Could you check a few things on this model? Use its own coordinates, in mm. A direction names the side the tool comes from. Round coordinates to 2 decimals unless told otherwise and drop trailing zeros. Write each loop counter-clockwise with the first axis right and the second up, starting at its lowest first coordinate (ties: lowest second). Pieces come first, ordered by that corner, then holes. Notation, with made-up numbers: M 67.25,25 L 94.25,25 A14 cw 94.25,38 Z; hole C -39,86 d11. An arc over 180 degrees is marked long. One line per item, written item: value. Start each with the question number.
(1) I want a section at C-C on x = -10. Please give me the cut outline in (y, z), and give its area (3 significant figures).
(2) I want a section at D-D on y = 20. Please give me the cut outline in (x, z).
(3) I want a section at B-B on y = 0. Please give me the cut outline in (x, z), and give its area (3 significant figures).
(4) Thinking about a two-plate mould opening in Y: for faces 4 (the face through (31, 9.76, 49.3)), 5 (the face through (162.942, 0, 50)), 6 (the face through (-121.037, -5.42, 74.406)), which applies, released by +Y, released by -Y, zero draft, split by the parting line, or undercut?
(5) I want a section at A-A on z = 17. Please give me the cut outline in (x, y), and give its area (3 significant figures).
(6) I'm going to push flat-ended pins straight in: pin 1 Ø1 at (x, y) = (-8.5, -41.5) entering from -Z; pin 2 Ø5 at (y, z) = (44.5, 53) entering from +X; pin 3 Ø10 at (y, z) = (-47, 45.5) entering from -X; pin 4 Ø10 at (x, z) = (-54.5, 81.5) entering from +Y. Where does each tip first touch, or does it pass through?
(7) Which directions (+Z, -Z, +X, -X, +Y, -Y) give clear straight access to the entire face, cutting with the end or side of a thin tool? Please do faces 1 (the face through (-77.942, 11, 27)), 2 (the face through (119.847, -5.42, 25.594)), 3 (the face through (-39.517, -67.185, 49.3)).
(8) If I drill on L1, parallel to Y at x = 0, z = 68; L2, parallel to Z at x = -141, y = -5.5; L3, parallel to Y at x = -83.5, z = 64.5, over which ranges is the centre line in solid material (lowest first)?
```python
from build123d import *

# Parameters (mm, degrees)
SKETCH1_R           = 32.5
BOSS_EXTRUDE1_DEPTH = 100
SKETCH2_R           = 25
BOSS_EXTRUDE2_DEPTH = 85
BOSS_EXTRUDE3_START = 85
SKETCH3_R           = 25
BOSS_EXTRUDE3_DEPTH = 85


with BuildPart() as part:
    # Sketch1 → Boss-Extrude1 (new body)
    with BuildSketch(Plane.XY):
        Polygon((0, -90), (77.942286341, -45), (77.942286341, 45), (0, 90), (-77.942286341, 45), (-77.942286341, -45), align=None)
        Circle(SKETCH1_R, mode=Mode.SUBTRACT)
    extrude(amount=BOSS_EXTRUDE1_DEPTH)

    # Sketch2 → Boss-Extrude2 (add)
    with BuildSketch(Plane(origin=(77.942286341, 0, 0), x_dir=(0, 0, -1), z_dir=(1, 0, 0))):
        with Locations(Location((-50, 0, 0), (0, 0, 90))):
            Circle(SKETCH2_R)
    extrude(amount=BOSS_EXTRUDE2_DEPTH)

    # Sketch3 → Boss-Extrude3 (add)
    with BuildSketch(Plane.ZY.offset(77.942286341).offset(BOSS_EXTRUDE3_START)):
        with Locations(Location((50, 0, 0), (0, 0, 90))):
            Circle(SKETCH3_R)
    extrude(amount=-BOSS_EXTRUDE3_DEPTH)


solid = part.part
```
Found:
1. outline: M -84.23,0 L -30.92,0 L -30.92,100 L -84.23,100 Z; M 30.92,0 L 84.23,0 L 84.23,100 L 30.92,100 Z
1. area: 10,700 mm²
2. outline: M -162.94,35 L -77.94,35 L -77.94,0 L -25.62,0 L -25.62,100 L -77.94,100 L -77.94,65 L -162.94,65 Z; M 25.62,0 L 77.94,0 L 77.94,35 L 162.94,35 L 162.94,65 L 77.94,65 L 77.94,100 L 25.62,100 Z
3. outline: M -162.94,25 L -77.94,25 L -77.94,0 L -32.5,0 L -32.5,100 L -77.94,100 L -77.94,75 L -162.94,75 Z; M 32.5,0 L 77.94,0 L 77.94,25 L 162.94,25 L 162.94,75 L 77.94,75 L 77.94,100 L 32.5,100 Z
3. area: 17,600 mm²
4. face 4: undercut
4. face 5: zero draft
4. face 6: split by the parting line
5. outline: M -77.94,-45 L 0,-90 L 77.94,-45 L 77.94,45 L 0,90 L -77.94,45 Z; hole C 0,0 d65
5. area: 17,700 mm²
6. pin 1: stops at z = 0
6. pin 2: stops at x = 77.94
6. pin 3: stops at x = -77.94
6. pin 4: stops at y = 61.42
7. face 1: -X
7. face 2: +X
7. face 3: +Z, -Z, -X, -Y
8. L1: y = -90 to -32.5, 32.5 to 90
8. L2: z = 25.61 to 74.39
8. L3: y = -20.37 to 20.37
